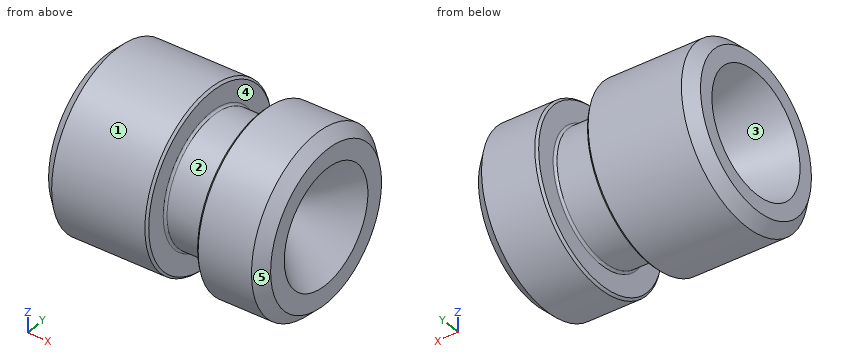
```python
from build123d import *

# Parameters (mm, degrees)
CHAMFER1_SIZE = 0.5
FILLET1_R     = 0.1
CHAMFER2_SIZE = 0.1


with BuildPart() as part:
    # Sketch1 → Revolve1 (revolve)
    with BuildSketch(Plane.XY):
        Polygon((-8, -2.743593539), (-8, -3.95), (-3.2, -3.95), (-3.2, -2.85), (-1, -2.85), (-1, -3.95), (2, -3.95), (2, -2.6), (0, -0.6), align=None)
    revolve(axis=Axis((-24.298547045, 0, 0), (1, 0, 0)))

    # Chamfer1
    chamfer1_edges = [part.edges().sort_by_distance(p)[0] for p in [
        (-8, 3.95, 0),
        (2, 3.95, 0),
    ]]
    chamfer(chamfer1_edges, length=CHAMFER1_SIZE)

    # Fillet1
    fillet1_edges = [part.edges().sort_by_distance(p)[0] for p in [
        (-1, 2.85, 0),
        (-3.2, 2.85, 0),
    ]]
    fillet(fillet1_edges, radius=FILLET1_R)

    # Chamfer2
    chamfer2_edges = [part.edges().sort_by_distance(p)[0] for p in [
        (-3.2, 3.95, 0),
        (-1, 3.95, 0),
    ]]
    chamfer(chamfer2_edges, length=CHAMFER2_SIZE)


solid = part.part
```
Check sheet for the modelled part. Datum: model origin and axes. Units: mm. Face numbers are marked on the shaded views. A direction names the side the tool comes from. Coordinates: 2 decimals unless noted, no trailing zeros. Loops run counter-clockwise (first coordinate to the right, second up) from the corner with the lowest first, then second, coordinate; pieces in that order, holes last.
1) Access from +Z, -Z, +X, -X, +Y, -Y to the whole of each face (thin tool, end or side, straight path). Record for the marked faces 1 and 2.
2) Sectioned sample at D-D (x = -2). Record the boundary of the cut face in (y, z).
3) Material ranges on probe 1 along X at (y, z) = (-0.5, 3); probe 2 along Y at (x, z) = (-5.25, 1.25); probe 3 along Z at (x, y) = (-6, -0.25), recorded low to high.
4) Sectioned sample at C-C (x = -4.75). Record the boundary of the cut face in (y, z).
5) Release check for a two-part mould opening along Z. For the marked faces 3, 4 and 5 record: released by +Z, released by -Z, zero draft, split by the parting line, or undercut.
6) Gauge pin test, flat ends, axial feed: pin 1 (1.5 mm diameter, centred on y = -1, z = 0.5, fed in from +X); pin 2 (1 mm diameter, centred on x = -6, z = 1.5, fed in from -Y); pin 3 (2 mm diameter, centred on x = -3.5, z = -1.5, fed in from +Y). Record the tip position at first contact, or that the pin passes through.
Check sheet entries:
1. face 1: +X, -X
1. face 2: none
2. outline: circle Ø5.7 at (0, 0); hole circle Ø2.27 at (0, 0)
3. probe 1: x = -8 to -3.2, -1 to 2
3. probe 2: y = -3.75 to -1.57, 1.57 to 3.75
3. probe 3: z = -3.94 to -2.19, 2.19 to 3.94
4. outline: circle Ø7.9 at (0, 0); hole circle Ø3.75 at (0, 0)
5. face 3: undercut
5. face 4: zero draft
5. face 5: split by the parting line
6. pin 1: stops at x = 1.27
6. pin 2: stops at y = -3.82
6. pin 3: stops at y = 3.92
